Input: dimensioned drawing with shaded views. Units: mm. Origin: part minimum x, y, z. Round coordinates to 2 decimals unless told otherwise and drop trailing zeros. Order: outer loops, then holes, each group sorted by start corner. A loop starts at its lowest first (then second) coordinate and runs counter-clockwise, first axis right, second up. Notation, with made-up numbers: M -12.5,70 L 36.5,70 A21 cw 36.5,91 Z; hole C 2,12.25 d5. An arc over 180 degrees is marked long. One line per question, with ' | ' between items.
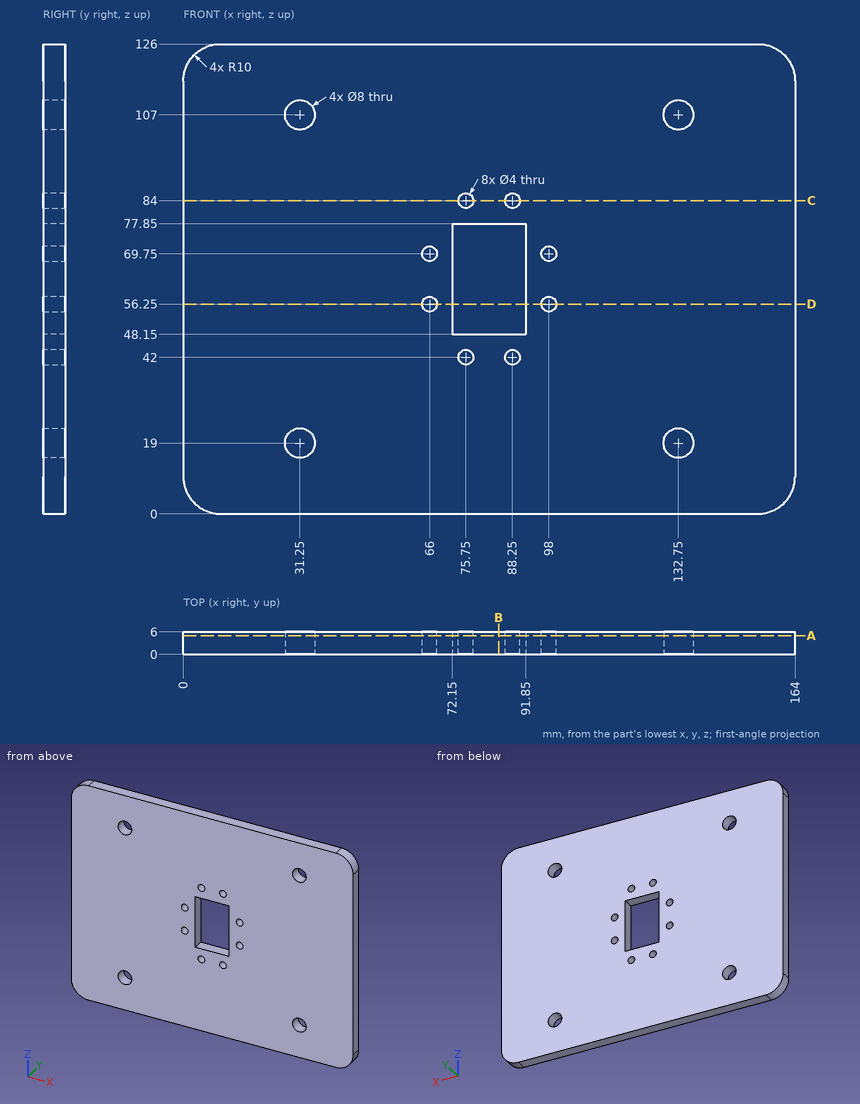
Item 1: Section query A-A, the plane y = 5. Give the number of separate pieces and of enclosed holes in the cut face, plus the area to 3 significant figures.
Report:
separate pieces: 1 | enclosed holes: 13 | area: 19,700 mm²
Item 2: Section query C-C, the plane z = 84. Return loops of the section in (x, y).
Report:
outline: M 0,0 L 73.75,0 L 73.75,6 L 0,6 Z; M 77.75,0 L 86.25,0 L 86.25,6 L 77.75,6 Z; M 90.25,0 L 164,0 L 164,6 L 90.25,6 Z
Item 3: Section query B-B, the plane x = 84.5. Return loops of the section in (y, z).
Report:
outline: M 0,0 L 6,0 L 6,48.15 L 0,48.15 Z; M 0,77.85 L 6,77.85 L 6,126 L 0,126 Z
Item 4: Line query: line 1 along X through (y, z) = (2.35, 84); line 2 along X through (y, z) = (2.25, 19); line 3 along Z through (x, y) = (133, 3.8). Output: solid intervals per line, ascending. Write a range as from..to.
Report:
line 1: 0..73.75, 77.75..86.25, 90.25..164 | line 2: 0..27.25, 35.25..128.75, 136.75..164 | line 3: 0..15.01, 22.99..103.01, 110.99..126
Item 5: Section query D-D, the plane z = 56.25. Return loops of the section in (x, y).
Report:
outline: M 0,0 L 64,0 L 64,6 L 0,6 Z; M 68,0 L 72.15,0 L 72.15,6 L 68,6 Z; M 91.85,0 L 96,0 L 96,6 L 91.85,6 Z; M 100,0 L 164,0 L 164,6 L 100,6 Z
